from build123d import *

# Parameters (mm, degrees)
F1_DEPTH = 65.532
F2_T     = -2.54


with BuildPart() as f1:
    # F0 (on Top) → F1 (new body)
    with BuildSketch(Plane.XY):
        with BuildLine():
            ThreePointArc((49.733212, -6.131827), (50.015562, -3.07169), (50.109797, 0))
            ThreePointArc((50.109797, 0), (50.015562, 3.07169), (49.733212, 6.131827))
            ThreePointArc((49.733212, 6.131827), (38.545584, 12.524219), (43.839211, 24.271697))
            ThreePointArc((43.839211, 24.271697), (40.539677, 29.453799), (36.630817, 34.193201))
            ThreePointArc((36.630817, 34.193201), (23.822481, 32.788832), (21.200121, 45.404257))
            ThreePointArc((21.200121, 45.404257), (15.484779, 47.657249), (9.536694, 49.193934))
            ThreePointArc((9.536694, 49.193934), (0, 40.529226), (-9.536694, 49.193934))
            ThreePointArc((-9.536694, 49.193934), (-15.484779, 47.657249), (-21.200121, 45.404257))
            ThreePointArc((-21.200121, 45.404257), (-20.210903, 43.060827), (-19.873228, 40.539677))
            ThreePointArc((-19.873228, 40.539677), (-26.060614, 31.580122), (-36.630817, 34.193201))
            ThreePointArc((-36.630817, 34.193201), (-40.539677, 29.453799), (-43.839211, 24.271697))
            ThreePointArc((-43.839211, 24.271697), (-39.645809, 20.738747), (-38.076678, 15.484779))
            ThreePointArc((-38.076678, 15.484779), (-41.661483, 8.012287), (-49.733212, 6.131827))
            ThreePointArc((-49.733212, 6.131827), (-50.109797, 0), (-49.733212, -6.131827))
            ThreePointArc((-49.733212, -6.131827), (-41.661483, -8.012287), (-38.076678, -15.484779))
            ThreePointArc((-38.076678, -15.484779), (-39.645809, -20.738747), (-43.839211, -24.271697))
            ThreePointArc((-43.839211, -24.271697), (-40.539677, -29.453799), (-36.630817, -34.193201))
            ThreePointArc((-36.630817, -34.193201), (-26.060614, -31.580122), (-19.873228, -40.539677))
            ThreePointArc((-19.873228, -40.539677), (-20.210903, -43.060827), (-21.200121, -45.404257))
            ThreePointArc((-21.200121, -45.404257), (-15.484779, -47.657249), (-9.536694, -49.193934))
            ThreePointArc((-9.536694, -49.193934), (0, -40.529226), (9.536694, -49.193934))
            ThreePointArc((9.536694, -49.193934), (15.484779, -47.657249), (21.200121, -45.404257))
            ThreePointArc((21.200121, -45.404257), (23.822481, -32.788832), (36.630817, -34.193201))
            ThreePointArc((36.630817, -34.193201), (40.539677, -29.453799), (43.839211, -24.271697))
            ThreePointArc((43.839211, -24.271697), (38.545584, -12.524219), (49.733212, -6.131827))
        make_face()
    extrude(amount=F1_DEPTH)

    # F2
    f2_openings = [f1.faces().sort_by_distance(p)[0] for p in [
        (0, 0, 65.532),
    ]]
    offset(amount=F2_T, openings=f2_openings)


solid = f1.part
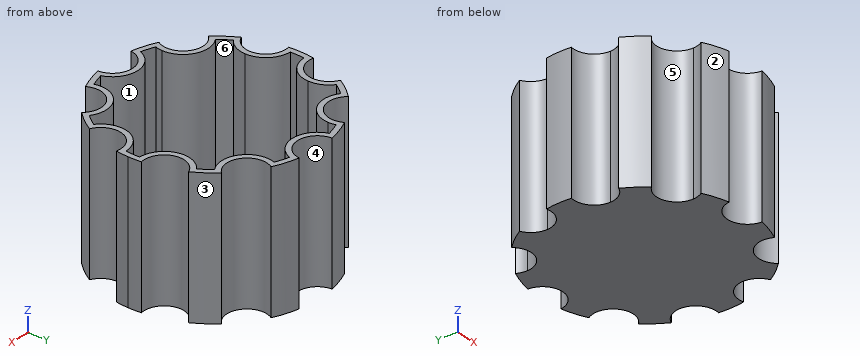
CAD build for the part. Positions are in the model's coordinates, mm. Face numbers are marked on the shaded views. A direction names the side the tool comes from. Coordinates: 2 decimals unless noted, no trailing zeros. Write each loop counter-clockwise with the first axis right and the second up, starting at its lowest first coordinate (ties: lowest second). Pieces come first, ordered by that corner, then holes. Notation, with made-up numbers: M -31,6.25 L 20,6.25 A18 cw 20,36.25 Z; hole C -33,66.5 d1. An arc over 180 degrees is marked long. Return JSON: item names as keys, results as strings.
Item 1: Slice it at B-B, the plane y = -23. Write the cut outline in (x, z), and give its area (3 significant figures).
Findings below:
{"outline": "M -41.72,0 L 41.72,0 L 41.72,65.53 L 38.15,65.53 L 38.15,2.54 L -38.15,2.54 L -38.15,65.53 L -41.72,65.53 Z", "area": "661 mm2"}
Item 2: Drop flat-ended pins along their axis: pin 1 Ø2 at (x, z) = (9.5, 40) entering from -Y; pin 2 Ø12 at (y, z) = (11, 24.5) entering from +X; pin 3 Ø1 at (y, z) = (12, 59) entering from +X; pin 4 Ø4 at (y, z) = (25.5, 8) entering from -X. Give the stop position or say it passes through.
Findings below:
{"pin 1": "stops at y = -49.19", "pin 2": "stops at x = 49.86", "pin 3": "stops at x = 38.94", "pin 4": "stops at x = -43.84"}
Item 3: Slice it at A-A, the plane x = -32. Write the cut outline in (y, z).
Findings below:
{"outline": "M -31.3,0 L 31.3,0 L 31.3,65.53 L 28.69,65.53 L 28.69,2.54 L -28.69,2.54 L -28.69,65.53 L -31.3,65.53 Z"}
Item 4: Probe line 1 (Y direction, x = -42, z = 58.5); line 2 (Y direction, x = 0.5, z = 34.5); line 3 (X direction, y = 40.5, z = 26.5). List the from-to ranges inside material, lowest first. Write a range as from..to.
Findings below:
{"line 1": "y = -27.33..-23.22, -7.75..-4.77, 4.77..7.75, 23.22..27.33", "line 2": "y = -40.54..-38, 38..40.54", "line 3": "x = -19.87..-17.33, -7.39..7.39, 17.33..19.87"}
Item 5: Two-plate mould, pull along Y, no slides. Class the marked faces 1, 2 and 3: +Y half, -Y half, draft (parallel to the pull), parting line (faces both ways), or undercut.
Findings below:
{"face 1": "undercut", "face 2": "-Y half", "face 3": "+Y half"}
Item 6: Which spindle directions (+Z, -Z, +X, -X, +Y, -Y) get a long thin tool onto all of the face, cutting with end or side? Do the marked faces 4, 5 and 6. Say none if no direction does.
Findings below:
{"face 4": "+Z, -Z, +Y", "face 5": "+Z, -Z", "face 6": "+Z"}
